The listing builds one solid part. Answer for the finished solid, in the listing's coordinates (mm). A direction names the side the tool comes from. Coordinates: 2 decimals unless noted, no trailing zeros. Write each loop counter-clockwise with the first axis right and the second up, starting at its lowest first coordinate (ties: lowest second). Pieces come first, ordered by that corner, then holes.
(1) The part is cut by section B-B on x = 0. Determine the outline of the cut face in (y, z), plus the area to 3 significant figures.
(2) Straight lines are drawn through the part: line 1 (Y direction, x = -5.5, z = 12); line 2 (Z direction, x = 0, y = 21). For each, find the intervals that lie inside material, in ascending order.
(3) For a pull along X with two mould halves and no side action, classify faces 4 (the flat face through (-20, -20, 30)), 5 (the flat face through (0, -10, 15)), 6 (the flat face through (25, 0, 10)), 7 (the cylindrical face through (-16.054, -18.757, 24.93)) as +X half, -X half, draft (parallel to the pull), parting line (faces both ways), or undercut.
(4) The part is cut by section A-A on z = 17.25. Determine the outline of the cut face in (x, y).
(5) The part is cut by section C-C on y = -7. Determine the outline of the cut face in (x, z), plus the area to 3 significant figures.
(6) Which of the six approach directions +Z, -Z, +X, -X, +Y, -Y give full straight-line access (tool end or side, diameter ignored) to faces 1 (the flat face through (0, 0, 0)), 2 (the flat face through (0, 10, 17)), 3 (the cylindrical face through (-0.54, 17.4, 11.56))?
(7) Given P1, Ø16, axis at x = 1.5, y = -5, coming from the +Z side; P2, Ø4.5, axis at x = 0, z = 14, coming from the +Y side, each flat-ended and moving along its own axis, determine where each tip first touches the part or whether it passes through.
(8) The part is cut by section D-D on z = 14. Determine the outline of the cut face in (x, y), plus the area to 4 significant figures.
from build123d import *

# Parameters (mm, degrees)
F0_W     = 50
F0_H     = 50
F1_DEPTH = 20
F2_W     = 20
F2_H     = 20
F3_DEPTH = 10
F4_R     = 4.13691
F5_DEPTH = 10
F6_R     = 2.5
F7_DEPTH = 24.5615


with BuildPart() as f1:
    # F0 (on Top) → F1 (new body)
    with BuildSketch(Plane.XY):
        Rectangle(F0_W, F0_H)
    extrude(amount=F1_DEPTH)

    # F2 (on face) → F3 (cut)
    with BuildSketch(Plane.XY.offset(20)):
        Rectangle(F2_W, F2_H)
    extrude(amount=-F3_DEPTH, mode=Mode.SUBTRACT)

    # F4 (on face) → F5 (join)
    with BuildSketch(Plane.XY.offset(20)):
        with Locations((-20, -20)):
            Circle(F4_R)
    extrude(amount=F5_DEPTH)

    # F6 (on face) → F7 (cut)
    with BuildSketch(Plane.XZ.offset(-10)):
        with Locations((0, 14)):
            Circle(F6_R)
    extrude(amount=-F7_DEPTH, mode=Mode.SUBTRACT)


solid = f1.part
Model answer:
1. outline: (-25, 0) - (25, 0) - (25, 11.5) - (10, 11.5) - (10, 10) - (-10, 10) - (-10, 20) - (-25, 20) - close; (10, 16.5) - (25, 16.5) - (25, 20) - (10, 20) - close
1. area: 725 mm2
2. line 1: y = -25 to -10, 10 to 25
2. line 2: z = 0 to 11.5, 16.5 to 20
3. face 4: draft
3. face 5: undercut
3. face 6: +X half
3. face 7: parting line
4. outline: (-25, -25) - (25, -25) - (25, 25) - (-25, 25) - close; hole (-10, -10) - (10, -10) - (10, 10) - (-10, 10) - close
5. outline: (-25, 0) - (25, 0) - (25, 20) - (10, 20) - (10, 10) - (-10, 10) - (-10, 20) - (-25, 20) - close
5. area: 800 mm2
6. face 1: -Z, +X, -X, +Y, -Y
6. face 2: +Z
6. face 3: +Y
7. P1: stops at z = 20
7. P2: stops at y = -10
8. outline: (-25, -25) - (25, -25) - (25, 25) - (2.5, 25) - (2.5, 10) - (10, 10) - (10, -10) - (-10, -10) - (-10, 10) - (-2.5, 10) - (-2.5, 25) - (-25, 25) - close
8. area: 2,025 mm2
